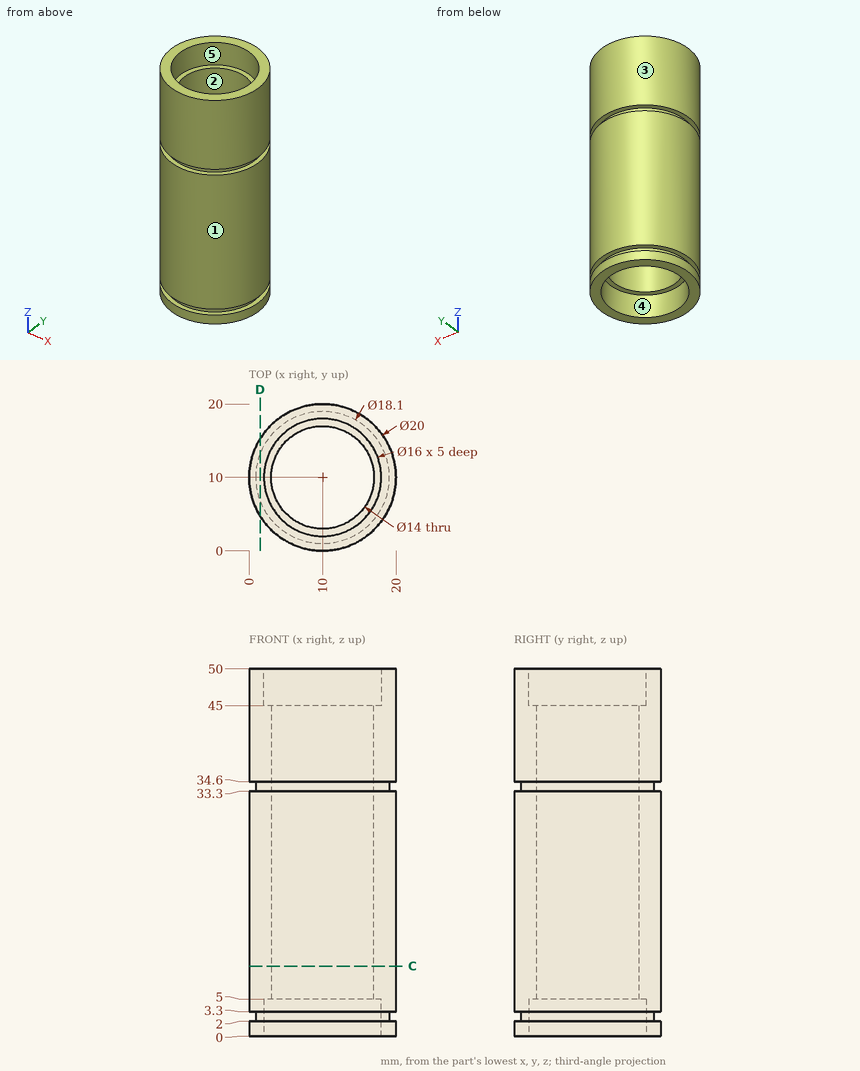
Geometry: see drawing. Coordinates: mm, zero at the bounding-box minimum. A direction names the side the tool comes from. Round coordinates to 2 decimals unless told otherwise and drop trailing zeros. Loops run counter-clockwise (first coordinate to the right, second up) from the corner with the lowest first, then second, coordinate; pieces in that order, holes last. Notation, with made-up numbers: (-1, 1) - (39, 1) arc R13 ccw to (39, 17) - close; hole circle Ø9 at (1.5, -20). An arc over 180 degrees is marked (long way). One line per item, written item: value. Start each with the question number.
(1) Contact query for flat-ended pins moving along their axis: P1, Ø5, axis at x = 14, z = 33.5, coming from the -Y side; P2, Ø5, axis at y = 8, z = 25.5, coming from the -X side; P3, Ø6, axis at y = 5.5, z = 36, coming from the +X side; P4, Ø1.5, axis at x = 5.5, y = 13, coming from the -Z side. Output: stop coordinate, or through.
(2) Section D-D, the plane x = 1.5. Return loops of the section in (y, z).
(3) Ray query, line 1 (Z direction, x = 16.75, y = 3.75); line 2 (Y direction, x = 10, z = 34); line 3 (Y direction, x = 10, z = 47.6). Return the intervals inside material, ascending. Write a range as [from, to].
(4) Section C-C, the plane z = 9.5. Return loops of the section in (x, y), plus the area to 3 significant figures.
(5) Access query for the marked faces 3, 4 and 5. Directions: +Z, -Z, +X, -X, +Y, -Y. A direction counts if a zero-diameter tool reaches every point of the face in a straight line with its end or side. Return the directions, or none.
(6) Draft query along X for the marked faces 1 and 2. Return one class per face: +X half, -X half, draft (parallel to the pull), parting line (faces both ways), or undercut.
Results below:
1. P1: y = 0.11
1. P2: x = 0
1. P3: x = 19.89
1. P4: through
2. outline: (4.73, 0) - (15.27, 0) - (15.27, 2) - (13.11, 2) - (13.11, 3.3) - (15.27, 3.3) - (15.27, 33.3) - (13.11, 33.3) - (13.11, 34.6) - (15.27, 34.6) - (15.27, 50) - (4.73, 50) - (4.73, 34.6) - (6.89, 34.6) - (6.89, 33.3) - (4.73, 33.3) - (4.73, 3.3) - (6.89, 3.3) - (6.89, 2) - (4.73, 2) - close
3. line 1: [0, 2], [3.3, 33.3], [34.6, 50]
3. line 2: [0.95, 3], [17, 19.05]
3. line 3: [0, 2], [18, 20]
4. outline: circle Ø20 at (10, 10); hole circle Ø14 at (10, 10)
4. area: 160 mm^2
5. face 3: +Z, -Z
5. face 4: -Z
5. face 5: +Z
6. face 1: parting line
6. face 2: undercut
